```python
from build123d import *

# Parameters (mm, degrees)
SKETCH_1_R               = 22.5
EXTRUDE_1_DEPTH          = 10.5
SKETCH_2_R               = 15
EXTRUDE_2_DEPTH          = 5
SKETCH_3_R               = 1.5
CUT_EXTRUDE_1_DEPTH      = 5
SKETCH_5_R               = 1.5
CUT_EXTRUDE_2_DEPTH      = 34.507461856
CUT_EXTRUDE_6_DEPTH      = 3
PATTERN_CIRCULAR_1_COUNT = 12
SKETCH_6_R               = 1.5
CUT_EXTRUDE_3_DEPTH      = 36.394208566
SKETCH_7_R               = 3
CUT_EXTRUDE_4_DEPTH      = 8
PATTERN_CIRCULAR_2_COUNT = 6
SKETCH_8_R               = 2
CUT_EXTRUDE_5_DEPTH      = 4
PATTERN_CIRCULAR_3_COUNT = 6


with BuildPart() as part:
    # 草图1 → 凸台-拉伸1 (new body)
    with BuildSketch(Plane.XY):
        with Locations(Location((0, 0, 0), (0, 0, 180))):
            Circle(SKETCH_1_R)
    extrude(amount=EXTRUDE_1_DEPTH)

    # 草图2 → 凸台-拉伸2 (add)
    with BuildSketch(Plane.XY.offset(10.5)):
        Circle(SKETCH_2_R)
    extrude(amount=EXTRUDE_2_DEPTH)

    # 草图3 → 切除-拉伸1 (cut)
    with BuildSketch(Plane.XY.offset(10.5)):
        with Locations((0, 18.5)):
            Circle(SKETCH_3_R)
    cut_extrude_1 = extrude(amount=-CUT_EXTRUDE_1_DEPTH, mode=Mode.SUBTRACT)

    # 草图5 → 切除-拉伸2 (cut, through all)
    with BuildSketch(Plane.XY.offset(10.5)):
        with Locations((0, 18.5)):
            Circle(SKETCH_5_R)
    cut_extrude_2 = extrude(amount=-CUT_EXTRUDE_2_DEPTH, mode=Mode.SUBTRACT)

    # 草图9 → 切除-拉伸6 (cut)
    with BuildSketch(Plane(origin=(0, 0, 0), x_dir=(-1, 0, 0), z_dir=(0, 0, -1))):
        Polygon((1.313991975, 21.705218415), (-2.118804585, 21.240559639), (-3.43279656, 18.035341223), (-1.313991975, 15.294781585), (2.118804585, 15.759440361), (3.43279656, 18.964658777), align=None)
    cut_extrude_6 = extrude(amount=-CUT_EXTRUDE_6_DEPTH, mode=Mode.SUBTRACT)

    # 阵列(圆周)1: 切除-拉伸1, 切除-拉伸2, 切除-拉伸6 ×12 about axis
    pattern_circular_1_axis = Axis((0, 0, 0), (0, 0, 1))
    add([cut_extrude_1.rotate(pattern_circular_1_axis, i * 360 / PATTERN_CIRCULAR_1_COUNT) for i in range(1, PATTERN_CIRCULAR_1_COUNT)], mode=Mode.SUBTRACT)
    add([cut_extrude_2.rotate(pattern_circular_1_axis, i * 360 / PATTERN_CIRCULAR_1_COUNT) for i in range(1, PATTERN_CIRCULAR_1_COUNT)], mode=Mode.SUBTRACT)
    add([cut_extrude_6.rotate(pattern_circular_1_axis, i * 360 / PATTERN_CIRCULAR_1_COUNT) for i in range(1, PATTERN_CIRCULAR_1_COUNT)], mode=Mode.SUBTRACT)

    # 草图6 → 切除-拉伸3 (cut, through all)
    with BuildSketch(Plane(origin=(0, 0, 0), x_dir=(-1, 0, 0), z_dir=(0, 0, -1))):
        with Locations((3.235238064, 12.074072829)):
            Circle(SKETCH_6_R)
    cut_extrude_3 = extrude(amount=-CUT_EXTRUDE_3_DEPTH, mode=Mode.SUBTRACT)

    # 草图7 → 切除-拉伸4 (cut)
    with BuildSketch(Plane.XY.offset(15.5)):
        with Locations((-3.235238064, 12.074072829)):
            Circle(SKETCH_7_R)
    cut_extrude_4 = extrude(amount=-CUT_EXTRUDE_4_DEPTH, mode=Mode.SUBTRACT)

    # 阵列(圆周)2: 切除-拉伸3, 切除-拉伸4 ×6 about axis
    pattern_circular_2_axis = Axis((0, 0, 0), (0, 0, 1))
    add([cut_extrude_3.rotate(pattern_circular_2_axis, i * 360 / PATTERN_CIRCULAR_2_COUNT) for i in range(1, PATTERN_CIRCULAR_2_COUNT)], mode=Mode.SUBTRACT)
    add([cut_extrude_4.rotate(pattern_circular_2_axis, i * 360 / PATTERN_CIRCULAR_2_COUNT) for i in range(1, PATTERN_CIRCULAR_2_COUNT)], mode=Mode.SUBTRACT)

    # 草图8 → 切除-拉伸5 (cut)
    with BuildSketch(Plane(origin=(0, 0, 0), x_dir=(-1, 0, 0), z_dir=(0, 0, -1))):
        with Locations((-2.63995426, 9.852443428)):
            Circle(SKETCH_8_R)
    cut_extrude_5 = extrude(amount=-CUT_EXTRUDE_5_DEPTH, mode=Mode.SUBTRACT)

    # 阵列(圆周)3: 切除-拉伸5 ×6 about axis
    pattern_circular_3_axis = Axis((0, 0, 0), (0, 0, 1))
    for i in range(1, PATTERN_CIRCULAR_3_COUNT):
        add(cut_extrude_5.rotate(pattern_circular_3_axis, i * 360 / PATTERN_CIRCULAR_3_COUNT), mode=Mode.SUBTRACT)


solid = part.part
```
Check sheet for the modelled part. Datum: model origin and axes. Units: mm. A direction names the side the tool comes from. Round coordinates to 2 decimals unless told otherwise and drop trailing zeros. Order: outer loops, then holes, each group sorted by start corner. A loop starts at its lowest first (then second) coordinate and runs counter-clockwise, first axis right, second up. Notation, with made-up numbers: (7, -34) - (20, -34) arc R15 cw to (20, -13) - close; hole circle Ø11 at (-26, -33). An arc over 180 degrees is marked (long way). Answer as CSV lines item,"result". Start each with the question number.
1) Scan lines: probe 1 along Y at (x, z) = (-0.5, 7); probe 2 along Y at (x, z) = (-10, 3.25); probe 3 along X at (y, z) = (-11, 1.25). Record each from-to range of solid material in increasing order.
2) Tool access check on faces 1 (the face through (9.825, -14.636, 6.802)), 2 (the face through (15, -11, 3)). Record the directions out of +Z, -Z, +X, -X, +Y, -Y that give a thin tool (end or side, any length) a straight path to the whole face; none if there is none.
3) Draft check along Y on faces 3 (the face through (18.41, 7.434, 1.479)), 4 (the face through (-10.382, 19.961, 5.176)). Enter one of: +Y half, -Y half, draft (parallel to the pull), parting line (faces both ways), or undercut.
4) Section check B-B (z = 4.75). Give the number of separate pieces and of enclosed holes in the cut face, then the cut area to 3 significant figures.
5) Depth check by flat-ended pin: pin 1 (3.5 mm diameter, centred on x = -9.85, y = -2.64, fed in from -Z); pin 2 (3 mm diameter, centred on y = -9.5, z = 10.5, fed in from +X); pin 3 (2 mm diameter, centred on y = 14.5, z = 9, fed in from -X); pin 4 (2.5 mm diameter, centred on x = 16.02, y = 9.25, fed in from -Z) (3 decimals). Enter the tip coordinate at first touch or a pass-through.
6) Section check A-A (z = 13.25). Record the cut outline in (x, y), then the cut area to 3 significant figures.
Determined:
1,probe 1,"-22.49 to -19.91, -17.09 to 17.09, 19.91 to 22.49"
1,probe 2,"-20.16 to -17.32, -14.72 to -9.79, -7.89 to -4.63, -0.65 to 14.72, 17.32 to 20.16"
1,probe 3,"-19.63 to -18.55, -13.58 to -4.28, -1 to 2.19, 4.28 to 13.5, 18.46 to 19.63"
2,face 1,"+Z, -Z"
2,face 2,"-Z"
3,face 3,"undercut"
3,face 4,"parting line"
4,separate pieces,"1"
4,enclosed holes,"18"
4,area,"1,460 mm^2"
5,pin 1,"z = 4"
5,pin 2,"x = 21.03"
5,pin 3,"x = -18"
5,pin 4,"through"
6,outline,"(-14.85, 2.1) arc R15 ccw to (-11.81, -9.25) arc R3 cw (long way) to (-9.25, -11.81) arc R15 ccw to (2.1, -14.85) arc R3 cw (long way) to (5.61, -13.91) arc R15 ccw to (13.91, -5.61) arc R3 cw (long way) to (14.85, -2.1) arc R15 ccw to (11.81, 9.25) arc R3 cw (long way) to (9.25, 11.81) arc R15 ccw to (-2.1, 14.85) arc R3 cw (long way) to (-5.61, 13.91) arc R15 ccw to (-13.91, 5.61) arc R3 cw (long way) to start"
6,area,"545 mm^2"
